Can you work these out from the model? Positions are in its coordinate system, mm. Face numbers are marked on the shaded views. A direction names the side the tool comes from. Coordinates: 2 decimals unless noted, no trailing zeros. Order: outer loops, then holes, each group sorted by start corner. A loop starts at its lowest first (then second) coordinate and runs counter-clockwise, first axis right, second up. Notation, with made-up numbers: M -2.5,80.25 L 6.5,80.25 A8 cw 6.5,84.25 Z; hole C 84.25,-2 d11. An arc over 180 degrees is marked long. Answer as a JSON object with one key per item and string values.
from build123d import *

# Parameters (mm, degrees)
EXTRUDE_1_DEPTH     = 7.9375
SKETCH_4_R          = 1.9
CUT_EXTRUDE_3_DEPTH = 19.796965347
SKETCH_5_R          = 3.2385
CUT_EXTRUDE_4_DEPTH = 19.796965347


with BuildPart() as part:
    # 草图1 → 凸台-拉伸1 (new body)
    with BuildSketch(Plane.XY):
        with BuildLine():
            Line((-5.08, 12.7), (-5.08, 5.679612663))
            ThreePointArc((-5.08, 5.679612663), (-7.62, 0), (-5.08, -5.679612663))
            Line((-5.08, -5.679612663), (-5.08, -12.7))
            ThreePointArc((-5.08, -12.7), (-4.336051224, -14.496051224), (-2.54, -15.24))
            Line((-2.54, -15.24), (2.54, -15.24))
            ThreePointArc((2.54, -15.24), (4.336051224, -14.496051224), (5.08, -12.7))
            Line((5.08, -12.7), (5.08, -5.679612663))
            ThreePointArc((5.08, -5.679612663), (7.62, 0), (5.08, 5.679612663))
            Line((5.08, 5.679612663), (5.08, 12.7))
            ThreePointArc((5.08, 12.7), (4.336051224, 14.496051224), (2.54, 15.24))
            Line((2.54, 15.24), (-2.54, 15.24))
            ThreePointArc((-2.54, 15.24), (-4.336051224, 14.496051224), (-5.08, 12.7))
        make_face()
    extrude(amount=EXTRUDE_1_DEPTH)

    # 草图4 → 切除-拉伸3 (cut, through all)
    with BuildSketch(Plane(origin=(0, 0, 0), x_dir=(-1, 0, 0), z_dir=(0, 0, -1))):
        with Locations((0, 10.922)):
            Circle(SKETCH_4_R)
    cut_extrude_3 = extrude(amount=-CUT_EXTRUDE_3_DEPTH, mode=Mode.SUBTRACT)

    # 镜向1: 切除-拉伸3 across plane
    add(cut_extrude_3.mirror(Plane.ZX), mode=Mode.SUBTRACT)

    # 草图5 → 切除-拉伸4 (cut, through all)
    with BuildSketch(Plane.XY.offset(7.9375)):
        Circle(SKETCH_5_R)
    extrude(amount=-CUT_EXTRUDE_4_DEPTH, mode=Mode.SUBTRACT)


solid = part.part
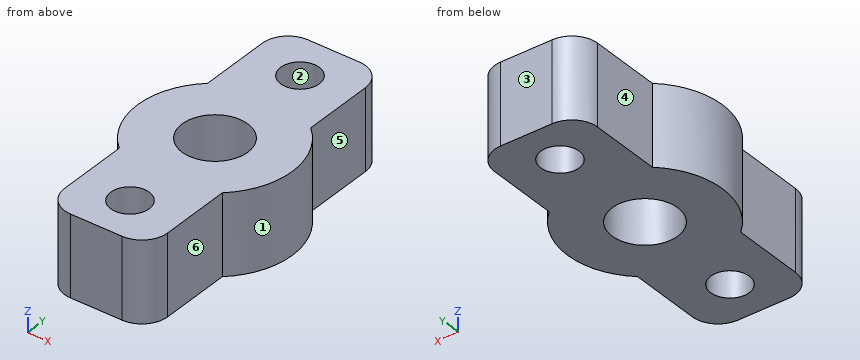
Item 1: I want a section at A-A, the plane y = 0. Write out the boundary of the cut face in (x, z), plus the area to 3 significant figures.
Answers follow:
{"outline": "M -7.62,0 L -3.24,0 L -3.24,7.94 L -7.62,7.94 Z; M 3.24,0 L 7.62,0 L 7.62,7.94 L 3.24,7.94 Z", "area": "69.6 mm^2"}
Item 2: If we mould it in two halves opening along X, with no side actions, what happens to the marked faces 1, 2 and 3? For each: pulls with the +X half, pulls with the -X half, needs draft (parallel to the pull), parting line crosses it, or undercut.
Answers follow:
{"face 1": "pulls with the +X half", "face 2": "undercut", "face 3": "needs draft"}
Item 3: I want a section at D-D, the plane y = -9.5. Write out the boundary of the cut face in (x, z), plus the area to 3 significant figures.
Answers follow:
{"outline": "M -5.08,0 L -1.26,0 L -1.26,7.94 L -5.08,7.94 Z; M 1.26,0 L 5.08,0 L 5.08,7.94 L 1.26,7.94 Z", "area": "60.6 mm^2"}
Item 4: I want a section at C-C, the plane z = 7. Write out the boundary of the cut face in (x, y).
Answers follow:
{"outline": "M -5.08,-12.7 A2.54 ccw -2.54,-15.24 L 2.54,-15.24 A2.54 ccw 5.08,-12.7 L 5.08,-5.68 A7.62 ccw 5.08,5.68 L 5.08,12.7 A2.54 ccw 2.54,15.24 L -2.54,15.24 A2.54 ccw -5.08,12.7 L -5.08,5.68 A7.62 ccw -5.08,-5.68 Z; hole C 0,0 d6.48; hole C 0,-10.92 d3.8; hole C 0,10.92 d3.8"}
Item 5: Which directions (+Z, -Z, +X, -X, +Y, -Y) give clear straight access to the entire face, cutting with the end or side of a thin tool? Please do the marked faces 4, 5 and 6.
Answers follow:
{"face 4": "+Z, -Z, -X, +Y", "face 5": "+Z, -Z, +X, +Y", "face 6": "+Z, -Z, +X, -Y"}
Item 6: Please list where these lines run through material, in increasing order: line 1 (Y direction, x = 0, z = 5.75); line 2 (X direction, y = 8.5, z = 4.75); line 3 (X direction, y = -9.5, z = 4).
Answers follow:
{"line 1": "y = -15.24 to -12.82, -9.02 to -3.24, 3.24 to 9.02, 12.82 to 15.24", "line 2": "x = -5.08 to 5.08", "line 3": "x = -5.08 to -1.26, 1.26 to 5.08"}
Item 7: I'm going to push flat-ended pins straight in: pin 1 (2 mm diameter, centred on y = 9, z = 5.5, fed in from -X); pin 2 (3.5 mm diameter, centred on x = 0, y = 10.922, fed in from +Z); pin 3 (4 mm diameter, centred on y = 9, z = 3, fed in from +X); pin 4 (2 mm diameter, centred on y = -5, z = 4, fed in from +X). Where does each tip first touch, or does it pass through?
Answers follow:
{"pin 1": "stops at x = -5.08", "pin 2": "passes through", "pin 3": "stops at x = 5.08", "pin 4": "stops at x = 6.49"}
Item 8: I want a section at B-B, the plane x = 0. Write out the boundary of the cut face in (y, z).
Answers follow:
{"outline": "M -15.24,0 L -12.82,0 L -12.82,7.94 L -15.24,7.94 Z; M -9.02,0 L -3.24,0 L -3.24,7.94 L -9.02,7.94 Z; M 3.24,0 L 9.02,0 L 9.02,7.94 L 3.24,7.94 Z; M 12.82,0 L 15.24,0 L 15.24,7.94 L 12.82,7.94 Z"}
